Could you check a few things on this model? Use its own coordinates, in mm. A direction names the side the tool comes from. Give positions to 0.01 mm unless a question says otherwise; leave off trailing zeros. Loops run counter-clockwise (first coordinate to the right, second up) from the corner with the lowest first, then second, coordinate; pieces in that order, holes last. Notation, with made-up numbers: (58, 51.5) - (74, 51.5) arc R20 ccw to (74, 55.5) - close; hole circle Ø7 at (-35.5, -22). An arc over 180 degrees is marked (long way). Answer in a Markdown table with one row per item. Add a question column.
Autodesk Fusion 360 part; units mm, degrees
sketch "Sketch1" plane through (0, 0, 0) normal (0, 0, 1) x (1, 0, 0)
  line L0 (4, 0) -> (0, 0)
  line L1 (0, 0) -> (0, 2.25)
  line L2 (0, 2.25) -> (1.5, 2.25)
  line L3 (1.5, 2.25) -> (1.5, 1.5)
  line L4 (1.5, 1.5) -> (2.75, 1.5)
  line L5 (2.75, 1.5) -> (2.75, 0.75)
  line L6 (2.75, 0.75) -> (4, 0.75)
  line L7 (4, 0.75) -> (4, 0)
  dimension "d1" = 4
  dimension "d4" = 2.25
  dimension "d5" = 1.25
  dimension "d6" = 1.5
  dimension "d7" = 0.75
  dimension "d8" = 0.75
  dimension "d10" = 1.25
sketch "Sketch2" plane through (0, 2.25, 0) normal (0, 1, 0) x (-1, 0, 0)
  line L0 (-1.5, 0) -> (0, 0)
  line L1 (0, 0) -> (0, 1.25)
  line L2 (0, 1.25) -> (-1.5, 1.25)
  line L3 (-1.5, 1.25) -> (-1.5, 0)
  line L4 (-1.5, 0.2963) -> (-0.6318, 0.2963)
  line L5 (-0.6318, 0.2963) -> (-0.6318, 0.976)
  line L6 (-0.6318, 0.976) -> (-3.3284, 0.976)
  line L7 (-3.3284, 0.976) -> (-3.3284, 0.2963)
  line L8 (-3.3284, 0.2963) -> (-1.5, 0.2963)
sketch "Sketch3" plane through (0, 0, 0) normal (0, 0, 1) x (1, 0, 0)
  line L0 (0, 0) -> (100, 0)
  line L1 (100, 0) -> (100, 40)
  line L2 (100, 40) -> (0, 40)
  line L3 (0, 40) -> (0, 0)
  dimension "d15" = 100
  dimension "d16" = 40
extrude "Extrude3" add sketch "Sketch3" along normal blind 60
sketch "Sketch4" plane through (0, 40, 0) normal (0, 1, 0) x (-1, 0, 0)
  line L0 (-100, 0) -> (0, 0)
  line L1 (0, 0) -> (0, 60)
  line L2 (0, 60) -> (-100, 60)
  line L3 (-100, 60) -> (-100, 0)
  line L4 (-20, 60) -> (-20, 20)
  line L5 (-20, 20) -> (-100, 20)
  dimension "d19" = 40
  dimension "d20" = 80
extrude "Extrude4" cut sketch "Sketch4" against normal blind 30 contours L2 L3 L4 L5
sketch "Sketch5" plane through (0, 40, 0) normal (0, 1, 0) x (-1, 0, 0)
  line L0 (-20, 60) -> (-20, 20)
  line L1 (-20, 20) -> (-100, 20)
  line L2 (-100, 20) -> (-100, 0)
  line L3 (-100, 0) -> (0, 0)
  line L4 (0, 0) -> (0, 60)
  line L5 (0, 60) -> (-20, 60)
  line L6 (-20, 40) -> (0, 40)
extrude "Extrude5" cut sketch "Sketch5" against normal blind 20 contours L0 L4 L5 L6
sketch "Sketch6" plane through (0, 40, 0) normal (0, 1, 0) x (-1, 0, 0)
  line L0 (0, 40) -> (-20, 40)
  line L1 (-20, 40) -> (-20, 20)
  line L2 (-20, 20) -> (-100, 20)
  line L3 (-100, 20) -> (-100, 0)
  line L4 (-100, 0) -> (0, 0)
  line L5 (0, 0) -> (0, 40)
  line L6 (-80, 0) -> (-80, 20)
extrude "Extrude6" cut sketch "Sketch6" against normal blind 10 contours L2 L3 L4 L6
(1) For pin 1 Ø22 at (x, y) = (11, 34) entering from +Z; pin 2 Ø6 at (x, z) = (92.5, 14.5) entering from +Y; pin 3 Ø8 at (y, z) = (35, 6.5) entering from +X, each with a flat end and sliding along its axis, tell me the tip position at first contact or that it passes through.
(2) I want a section at B-B on z = 30. Please give me the cut outline in (x, y), then the cut area to 3 significant figures.
(3) Please list where these lines run through material, in increasing order: line 1 (Y direction, x = 77.5, z = 35); line 2 (Z direction, x = 5, y = 37); line 3 (Z direction, x = 66, y = 16.5).
(4) I want a section at A-A on x = 50. Please give me the cut outline in (y, z), then the cut area to 3 significant figures.
(5) On a 3-axis mill with a long thin cutter (end or side, diameter ignored), from which of +Z, -Z, +X, -X, +Y, -Y can I reach the whole of each face in a straight line? I mean faces 1 (the flat face through (80, 35, 10)), 2 (the flat face through (10, 30, 40)), 3 (the flat face through (0, 20, 23)), 4 (the flat face through (59, 25, 20)), 5 (the flat face through (49, 0, 30)). Say none if no direction works.
Reported:
| question | item | result |
|---|---|---|
| 1 | pin 1 | z = 40 |
| 1 | pin 2 | y = 30 |
| 1 | pin 3 | x = 80 |
| 2 | outline | (0, 0) - (100, 0) - (100, 10) - (20, 10) - (20, 40) - (0, 40) - close |
| 2 | area | 1,600 mm² |
| 3 | line 1 | 0 to 10 |
| 3 | line 2 | 0 to 40 |
| 3 | line 3 | 0 to 20 |
| 4 | outline | (0, 0) - (40, 0) - (40, 20) - (10, 20) - (10, 60) - (0, 60) - close |
| 4 | area | 1,200 mm² |
| 5 | face 1 | +Z, -Z, +X, +Y |
| 5 | face 2 | +Z, +X, -X, +Y |
| 5 | face 3 | +Z, -Z, -X, +Y, -Y |
| 5 | face 4 | +Z, +X, +Y |
| 5 | face 5 | +Z, -Z, +X, -X, -Y |
